Verification items for the finished model (mm, model axes). Round coordinates to 2 decimals unless told otherwise and drop trailing zeros.
```python
from build123d import *

# Parameters (mm, degrees)
F0_R     = 2.15
F1_DEPTH = 250


# Not quite as in the source:
# - ends of sketch curves that miss each other by under 0.0002 mm in the source are joined


with BuildPart() as f1:
    # F0 (on Front) → F1 (new body, symmetric)
    with BuildSketch(Plane.XZ):
        with BuildLine():
            Line((7.5, 8.5), (7.5, 9.2))
            ThreePointArc((7.5, 9.2), (7.2656854249, 9.7656854249), (6.7, 10))
            Line((6.7, 10), (-6.7, 10))
            ThreePointArc((-6.7, 10), (-7.2656854249, 9.7656854249), (-7.5, 9.2))
            Line((-7.5, 9.2), (-7.5, 8.5))
            ThreePointArc((-7.5, 8.5), (-7.4121320344, 8.2878679656), (-7.2, 8.2))
            Line((-7.2, 8.2), (-5.004162, 8.2))
            ThreePointArc((-5.004162, 8.2), (-4.2650582387, 7.7061464193), (-4.4384770751, 6.8343140751))
            Line((-4.4384770751, 6.8343140751), (-6.744114, 4.528679))
            ThreePointArc((-6.744114, 4.528679), (-7.7173840295, 3.8783612672), (-8.865434, 3.65))
            Line((-8.865434, 3.65), (-11.134566, 3.65))
            ThreePointArc((-11.134566, 3.65), (-12.2826159705, 3.8783612672), (-13.2558858436, 4.5286791564))
            Line((-13.2558858436, 4.5286791564), (-15.561523, 6.834314))
            ThreePointArc((-15.561523, 6.834314), (-15.7349417613, 7.7061464193), (-14.995838, 8.2))
            Line((-14.995838, 8.2), (-12.8, 8.2))
            ThreePointArc((-12.8, 8.2), (-12.5878679656, 8.2878679656), (-12.5, 8.5))
            Line((-12.5, 8.5), (-12.5, 9.2))
            ThreePointArc((-12.5, 9.2), (-12.7343145751, 9.7656854249), (-13.3, 10))
            Line((-13.3, 10), (-18, 10))
            ThreePointArc((-18, 10), (-19.4142135624, 9.4142135624), (-20, 8))
            Line((-20, 8), (-20, 3.3))
            ThreePointArc((-20, 3.3), (-19.7656854249, 2.7343145751), (-19.2, 2.5))
            Line((-19.2, 2.5), (-18.500003, 2.5))
            ThreePointArc((-18.500003, 2.5), (-18.2878709656, 2.5878679656), (-18.200003, 2.8))
            Line((-18.200003, 2.8), (-18.200003, 4.995834))
            ThreePointArc((-18.200003, 4.995834), (-17.7061497459, 5.734937626), (-16.8343175751, 5.5615194249))
            Line((-16.8343175751, 5.5615194249), (-14.528682, 3.255884))
            ThreePointArc((-14.528682, 3.255884), (-13.8783635378, 2.2826136237), (-13.650002, 1.134563))
            Line((-13.650002, 1.134563), (-13.650002, -1.134563))
            ThreePointArc((-13.650002, -1.134563), (-13.8783635378, -2.2826136237), (-14.5286821564, -3.2558838436))
            Line((-14.5286821564, -3.2558838436), (-16.834318, -5.561519))
            ThreePointArc((-16.834318, -5.561519), (-17.7061497459, -5.734937626), (-18.200003, -4.995834))
            Line((-18.200003, -4.995834), (-18.200003, -2.8))
            ThreePointArc((-18.200003, -2.8), (-18.2878709656, -2.5878679656), (-18.500003, -2.5))
            Line((-18.500003, -2.5), (-19.2, -2.5))
            ThreePointArc((-19.2, -2.5), (-19.7656854249, -2.7343145751), (-20, -3.3))
            Line((-20, -3.3), (-20, -8))
            ThreePointArc((-20, -8), (-19.4142135624, -9.4142135624), (-18, -10))
            Line((-18, -10), (-13.3, -10))
            ThreePointArc((-13.3, -10), (-12.7343145751, -9.7656854249), (-12.5, -9.2))
            Line((-12.5, -9.2), (-12.5, -8.5))
            ThreePointArc((-12.5, -8.5), (-12.5878679656, -8.2878679656), (-12.8, -8.2))
            Line((-12.8, -8.2), (-14.995838, -8.2))
            ThreePointArc((-14.995838, -8.2), (-15.7349417613, -7.7061464193), (-15.5615229249, -6.8343140751))
            Line((-15.5615229249, -6.8343140751), (-13.255886, -4.528679))
            ThreePointArc((-13.255886, -4.528679), (-12.2826159705, -3.8783612672), (-11.134566, -3.65))
            Line((-11.134566, -3.65), (-8.865434, -3.65))
            ThreePointArc((-8.865434, -3.65), (-7.7173840295, -3.8783612672), (-6.7441141564, -4.5286791564))
            Line((-6.7441141564, -4.5286791564), (-4.438477, -6.834314))
            ThreePointArc((-4.438477, -6.834314), (-4.2650582387, -7.7061464193), (-5.004162, -8.2))
            Line((-5.004162, -8.2), (-7.2, -8.2))
            ThreePointArc((-7.2, -8.2), (-7.4121320344, -8.2878679656), (-7.5, -8.5))
            Line((-7.5, -8.5), (-7.5, -9.2))
            ThreePointArc((-7.5, -9.2), (-7.2656854249, -9.7656854249), (-6.7, -10))
            Line((-6.7, -10), (6.7, -10))
            ThreePointArc((6.7, -10), (7.2656854249, -9.7656854249), (7.5, -9.2))
            Line((7.5, -9.2), (7.5, -8.5))
            ThreePointArc((7.5, -8.5), (7.4121320344, -8.2878679656), (7.2, -8.2))
            Line((7.2, -8.2), (5.004162, -8.2))
            ThreePointArc((5.004162, -8.2), (4.2650582387, -7.7061464193), (4.4384770751, -6.8343140751))
            Line((4.4384770751, -6.8343140751), (6.744114, -4.528679))
            ThreePointArc((6.744114, -4.528679), (7.7173840295, -3.8783612672), (8.865434, -3.65))
            Line((8.865434, -3.65), (11.134566, -3.65))
            ThreePointArc((11.134566, -3.65), (12.2826159705, -3.8783612672), (13.2558858436, -4.5286791564))
            Line((13.2558858436, -4.5286791564), (15.561523, -6.834314))
            ThreePointArc((15.561523, -6.834314), (15.7349417613, -7.7061464193), (14.995838, -8.2))
            Line((14.995838, -8.2), (12.8, -8.2))
            ThreePointArc((12.8, -8.2), (12.5878679656, -8.2878679656), (12.5, -8.5))
            Line((12.5, -8.5), (12.5, -9.2))
            ThreePointArc((12.5, -9.2), (12.7343145751, -9.7656854249), (13.3, -10))
            Line((13.3, -10), (18, -10))
            ThreePointArc((18, -10), (19.4142135624, -9.4142135624), (20, -8))
            Line((20, -8), (20, -3.3))
            ThreePointArc((20, -3.3), (19.7656854249, -2.7343145751), (19.2, -2.5))
            Line((19.2, -2.5), (18.500003, -2.5))
            ThreePointArc((18.500003, -2.5), (18.2878709656, -2.5878679656), (18.200003, -2.8))
            Line((18.200003, -2.8), (18.200003, -4.995834))
            ThreePointArc((18.200003, -4.995834), (17.7061497459, -5.734937626), (16.8343175751, -5.5615194249))
            Line((16.8343175751, -5.5615194249), (14.528682, -3.255884))
            ThreePointArc((14.528682, -3.255884), (13.8783635378, -2.2826136237), (13.650002, -1.134563))
            Line((13.650002, -1.134563), (13.650002, 1.134563))
            ThreePointArc((13.650002, 1.134563), (13.8783635378, 2.2826136237), (14.5286821564, 3.2558838436))
            Line((14.5286821564, 3.2558838436), (16.834318, 5.561519))
            ThreePointArc((16.834318, 5.561519), (17.7061497459, 5.734937626), (18.200003, 4.995834))
            Line((18.200003, 4.995834), (18.200003, 2.8))
            ThreePointArc((18.200003, 2.8), (18.2878709656, 2.5878679656), (18.500003, 2.5))
            Line((18.500003, 2.5), (19.2, 2.5))
            ThreePointArc((19.2, 2.5), (19.7656854249, 2.7343145751), (20, 3.3))
            Line((20, 3.3), (20, 8))
            ThreePointArc((20, 8), (19.4142135624, 9.4142135624), (18, 10))
            Line((18, 10), (13.3, 10))
            ThreePointArc((13.3, 10), (12.7343145751, 9.7656854249), (12.5, 9.2))
            Line((12.5, 9.2), (12.5, 8.5))
            ThreePointArc((12.5, 8.5), (12.5878679656, 8.2878679656), (12.8, 8.2))
            Line((12.8, 8.2), (14.995838, 8.2))
            ThreePointArc((14.995838, 8.2), (15.7349417613, 7.7061464193), (15.5615229249, 6.8343140751))
            Line((15.5615229249, 6.8343140751), (13.255886, 4.528679))
            ThreePointArc((13.255886, 4.528679), (12.2826159705, 3.8783612672), (11.134566, 3.65))
            Line((11.134566, 3.65), (8.865434, 3.65))
            ThreePointArc((8.865434, 3.65), (7.7173840295, 3.8783612672), (6.7441141564, 4.5286791564))
            Line((6.7441141564, 4.5286791564), (4.438477, 6.834314))
            ThreePointArc((4.438477, 6.834314), (4.2650582387, 7.7061464193), (5.004162, 8.2))
            Line((5.004162, 8.2), (7.2, 8.2))
            ThreePointArc((7.2, 8.2), (7.4121320344, 8.2878679656), (7.5, 8.5))
        make_face()
        with Locations((-10, 0)):
            Circle(F0_R, mode=Mode.SUBTRACT)
        with BuildLine():
            ThreePointArc((-1.4142130624, 7.3129870624), (0, 7.898773), (1.4142130624, 7.3129870624))
            Line((1.4142130624, 7.3129870624), (5.471318, 3.255884))
            ThreePointArc((5.471318, 3.255884), (6.1216364622, 2.2826136237), (6.349998, 1.134563))
            Line((6.349998, 1.134563), (6.349998, -1.134563))
            ThreePointArc((6.349998, -1.134563), (6.1216364622, -2.2826136237), (5.4713178436, -3.2558838436))
            Line((5.4713178436, -3.2558838436), (1.414213, -7.312987))
            ThreePointArc((1.414213, -7.312987), (0, -7.898773), (-1.4142130624, -7.3129870624))
            Line((-1.4142130624, -7.3129870624), (-5.471318, -3.255884))
            ThreePointArc((-5.471318, -3.255884), (-6.1216364622, -2.2826136237), (-6.349998, -1.134563))
            Line((-6.349998, -1.134563), (-6.349998, 1.134563))
            ThreePointArc((-6.349998, 1.134563), (-6.1216364622, 2.2826136237), (-5.4713178436, 3.2558838436))
            Line((-5.4713178436, 3.2558838436), (-1.4142130624, 7.3129870624))
        make_face(mode=Mode.SUBTRACT)
        with Locations((10, 0)):
            Circle(F0_R, mode=Mode.SUBTRACT)
    extrude(amount=F1_DEPTH, both=True)


solid = f1.part
```
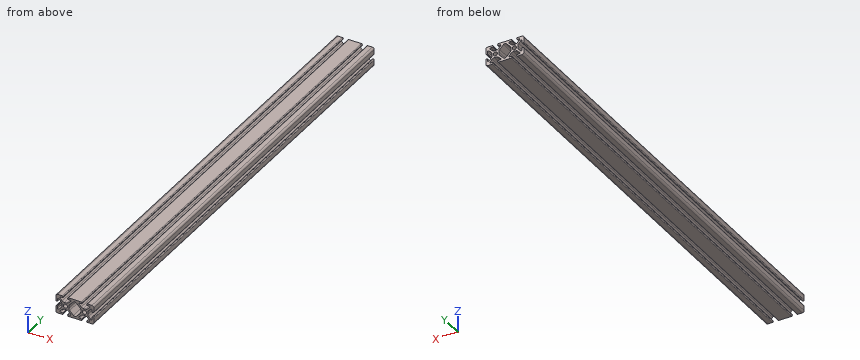
1) Sectioned sample at A-A on y = 145.5. Count the separate pieces of the cut face and the enclosed holes in it, then the cut area to 3 significant figures.
2) Scan lines: probe 1 along X at (y, z) = (154, -8.5); probe 2 along Z at (x, y) = (-15.5, -47.5); probe 3 along Z at (x, y) = (-13.5, -124.5). Record each from-to range of solid material in increasing order.
3) Go/stop test with flat-tipped pins: pin 1 Ø0.6 at (y, z) = (-74.5, -9) entering from -X; pin 2 Ø10 at (x, y) = (-8, 33) entering from -Z; pin 3 Ø0.7 at (y, z) = (115, 0.5) entering from +X; pin 4 Ø1.1 at (x, y) = (9.5, 92.5) entering from -Z. Record where each tip stops, or that it passes through.
Returned:
1. separate pieces: 1
1. enclosed holes: 3
1. area: 331 mm2
2. probe 1: x = -19.94 to -12.5, -7.5 to 7.5, 12.5 to 19.94
2. probe 2: z = -10 to -8.02, -6.77 to -4.23, 4.23 to 6.77, 8.02 to 10
2. probe 3: z = -10 to -8.2, -4.77 to 4.77, 8.2 to 10
3. pin 1: stops at x = -19.87
3. pin 2: stops at z = -10
3. pin 3: stops at x = 13.65
3. pin 4: stops at z = -3.65
